Answer from the drawing. Dimensions are ordinates in mm from the lowest x, y and z of the part. A direction names the side the tool comes from. Give positions to 0.01 mm unless a question says otherwise; leave off trailing zeros. Write each loop counter-clockwise with the first axis right and the second up, starting at its lowest first coordinate (ties: lowest second). Pieces come first, ordered by that corner, then holes. Notation, with made-up numbers: (82, 51.5) -> (109, 51.5) arc R19 cw to (109, 63.5) -> close; hole circle Ø11 at (-3.5, 12.25). An arc over 180 degrees is marked (long way). Use a Markdown table: item, result. Add a question column.
Q1. Each of these flat-tipped pins is pushed along its axis until it touches: pin 1 Ø1.5 at (y, z) = (84, 46.5) entering from -X (1 decimal); pin 2 Ø6 at (x, y) = (126, 89) entering from +Z. Where does it stop, or does it pass through?
Q2. Consider line 1 (X direction, y = 51.5, z = 13.5); line 2 (Y direction, x = 112.5, z = 5); line 3 (X direction, y = 86, z = 10) (1 decimal). Determine where each line is inside the solid, lowest interval first.
Q3. Section A-A, the plane y = 69 is taken. Give the vertices of the cut face in (x, z) (1 decimal).
Q4. For the marked faces 1, 2 and 3, determine the directions among +Z, -Z, +X, -X, +Y, -Y from which every point of the face is accessible in a straight line to the end or side of a thin tool.
Q5. For a pull along X with two mould halves and no side action, classify the marked faces 4, 5, 6 and 7 as pulls with the +X half, pulls with the -X half, needs draft (parallel to the pull), parting line crosses it, or undercut.
Q6. Section B-B, the plane y = 9 is taken. Give the vertices of the cut face in (x, z) (1 decimal), plus the area to 3 significant figures.
Q7. Section C-C, the plane x = 133.5 is taken. Give the vertices of the cut face in (y, z) (1 decimal).
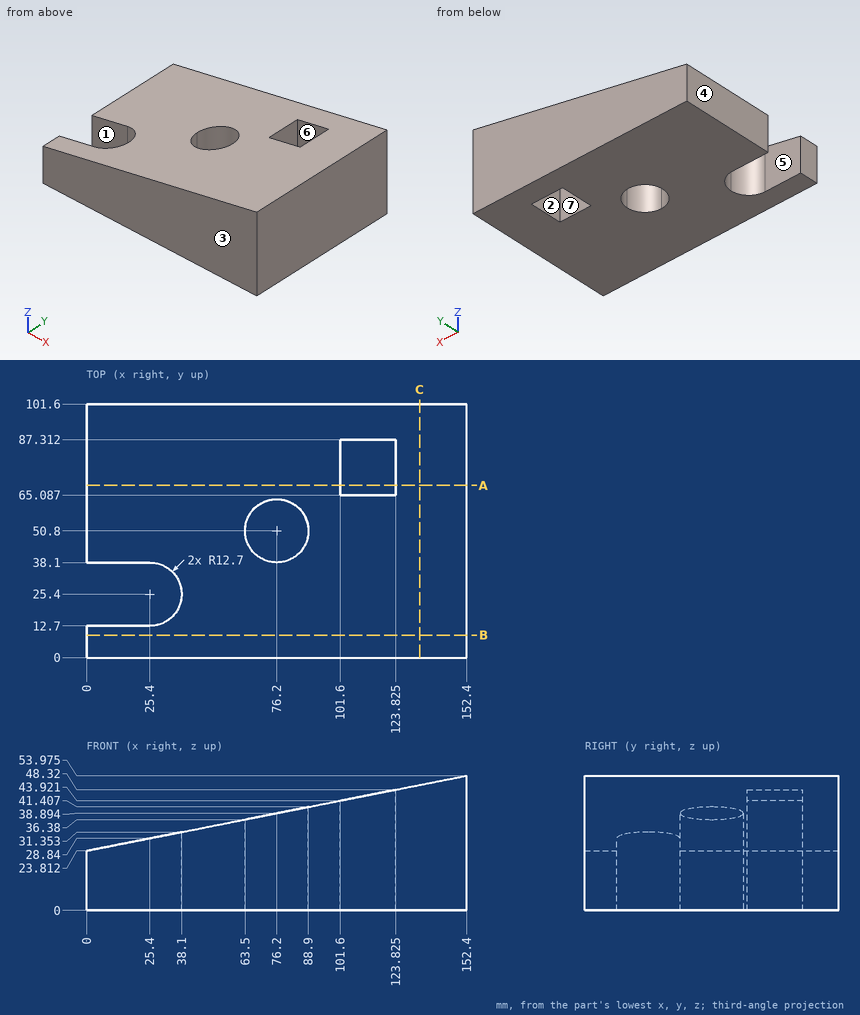
Result set:
| question | item | result |
|---|---|---|
| 1 | pin 1 | stops at x = 123.8 |
| 1 | pin 2 | stops at z = 49.34 |
| 2 | line 1 | x = 0 to 63.52, 88.88 to 152.4 |
| 2 | line 2 | y = 0 to 65.09, 87.31 to 101.6 |
| 2 | line 3 | x = 0 to 101.6, 123.8 to 152.4 |
| 3 | outline | (0, 0) -> (101.6, 0) -> (101.6, 43.9) -> (0, 23.8) -> close; (123.8, 0) -> (152.4, 0) -> (152.4, 54) -> (123.8, 48.3) -> close |
| 4 | face 1 | +Z, -Z, -X |
| 4 | face 2 | +Z, -Z |
| 4 | face 3 | +Z, -Z, +X, -X, -Y |
| 5 | face 4 | pulls with the -X half |
| 5 | face 5 | needs draft |
| 5 | face 6 | undercut |
| 5 | face 7 | undercut |
| 6 | outline | (0, 0) -> (152.4, 0) -> (152.4, 54) -> (0, 23.8) -> close |
| 6 | area | 5,930 mm2 |
| 7 | outline | (0, 0) -> (101.6, 0) -> (101.6, 50.2) -> (0, 50.2) -> close |
